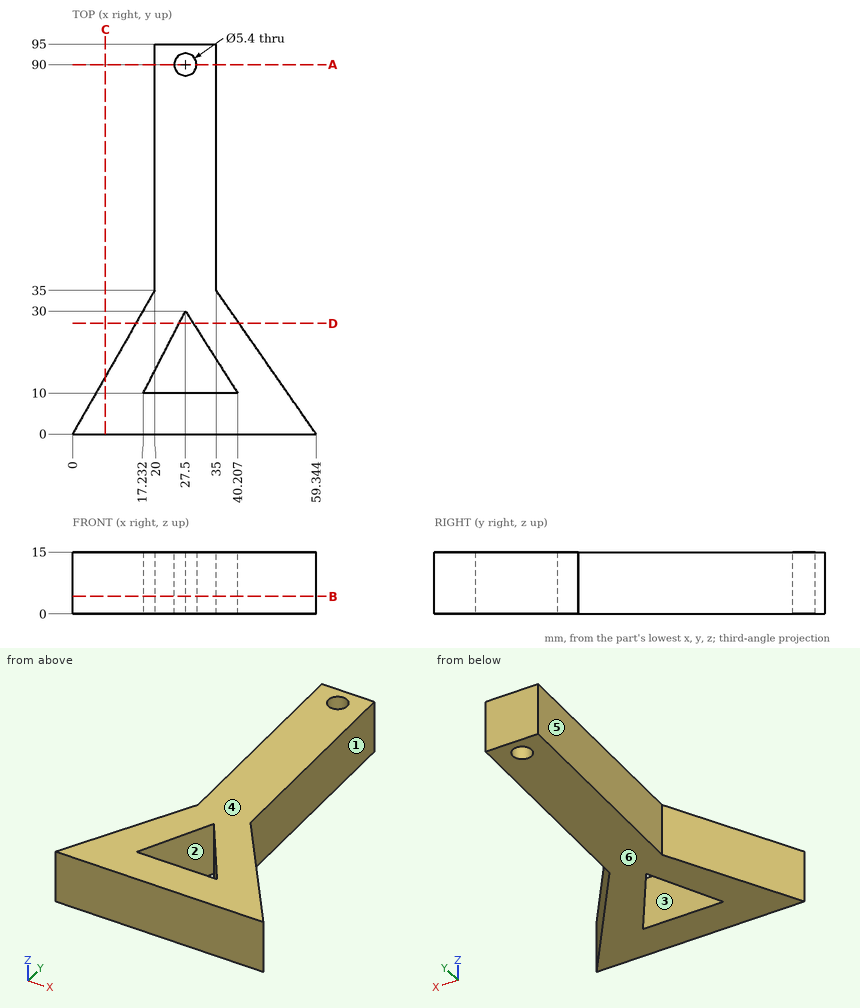
Study the drawing (mm; zero at the part's minimum x, y, z) and answer. A direction names the side the tool comes from. Give positions to 0.01 mm unless a question says otherwise; leave off trailing zeros. Order: outer loops, then holes, each group sorted by start corner. A loop starts at its lowest first (then second) coordinate and runs counter-clockwise, first axis right, second up. Notation, with made-up numbers: (-36.5, 46) - (-2.5, 46) arc R9 cw to (-2.5, 53) - close; hole circle Ø1 at (25, 60.25). An arc over 180 degrees is marked (long way). Use one line per item in the form item = value. Start each with the question number.
(1) Consider line 1 (X direction, y = 90, z = 5.5); line 2 (X direction, y = 51.5, z = 14); line 3 (X direction, y = 23.5, z = 7.5). Determine where each line is inside the solid, lowest interval first. Write a range as from..to.
(2) A cutting plane is placed at B-B, the plane z = 4.25. Write down the section's boundary in (x, y).
(3) Flat-ended cylindrical pins translate along their axes: pin 1 Ø2 at (y, z) = (77, 13.5) entering from +X; pin 2 Ø7 at (x, y) = (27.5, 90) entering from -Z; pin 3 Ø4.5 at (y, z) = (53, 9) entering from -X. Find the tip coordinate at first contact, or state that the pin passes through.
(4) For the marked faces 5 and 6, determine the directions among +Z, -Z, +X, -X, +Y, -Y from which every point of the face is accessible in a straight line to the end or side of a thin tool.
(5) A cutting plane is placed at D-D, the plane y = 27. Write down the section's boundary in (x, z) (1 decimal), then the cut area to 3 significant figures.
(6) The mould has two halves that part along X. Classify the marked faces 1, 2, 3 and 4: released by +X, released by -X, zero draft, split by the parting line, or undercut.
(7) A cutting plane is placed at C-C, the plane x = 8. Write down the section's boundary in (y, z).
(8) A cutting plane is placed at A-A, the plane y = 90. Write down the section's boundary in (x, z).
Ans:
q1.line_1 = 20..24.8, 30.2..35
q1.line_2 = 20..35
q1.line_3 = 13.43..24.16, 31.63..43
q2.outline = (0, 0) - (59.34, 0) - (35, 35) - (35, 95) - (20, 95) - (20, 35) - close; hole (17.23, 10) - (40.21, 10) - (27.5, 30) - close; hole circle Ø5.4 at (27.5, 90)
q3.pin_1 = 35
q3.pin_2 = 0
q3.pin_3 = 20
q4.face_5 = +Z, -Z, -X, +Y
q4.face_6 = -Z, +X, -X, +Y, -Y
q5.outline = (15.4, 0) - (26, 0) - (26, 15) - (15.4, 15) - close; (29.4, 0) - (40.6, 0) - (40.6, 15) - (29.4, 15) - close
q5.area = 325 mm^2
q6.face_1 = released by +X
q6.face_2 = undercut
q6.face_3 = undercut
q6.face_4 = zero draft
q7.outline = (0, 0) - (14, 0) - (14, 15) - (0, 15) - close
q8.outline = (20, 0) - (24.8, 0) - (24.8, 15) - (20, 15) - close; (30.2, 0) - (35, 0) - (35, 15) - (30.2, 15) - close
